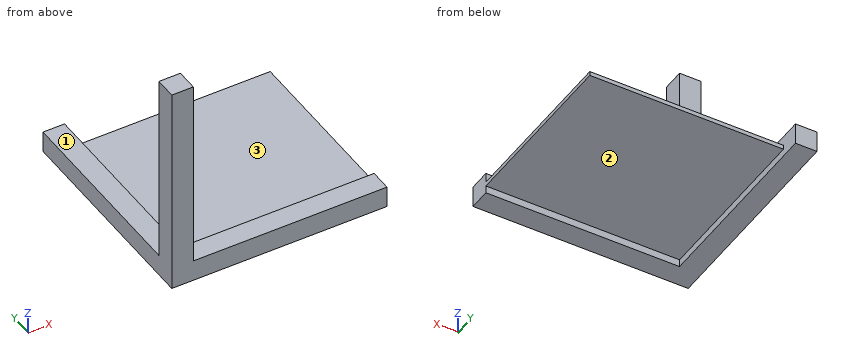
```python
from build123d import *

# Parameters (mm, degrees)
F0_W     = 200
F0_H     = 20
F1_DEPTH = 20
F2_W     = 20
F2_H     = 20
F3_DEPTH = 180
F4_W     = 20
F4_H     = 20
F5_DEPTH = 180
F6_W     = 180
F6_H     = 4
F7_DEPTH = 161.4


with BuildPart() as f1:
    # F0 (on Top) → F1 (new body)
    with BuildSketch(Plane.XY):
        with Locations((100, 10)):
            Rectangle(F0_W, F0_H)
    extrude(amount=F1_DEPTH)

    # F2 (on face) → F3 (join)
    with BuildSketch(Plane.XY.offset(20)):
        with Locations((10, 10)):
            Rectangle(F2_W, F2_H)
    extrude(amount=F3_DEPTH)

    # F4 (on face) → F5 (join)
    with BuildSketch(Plane(origin=(0, 20, 0), x_dir=(-1, 0, 0), z_dir=(0, 1, 0))):
        with Locations((-10, 10)):
            Rectangle(F4_W, F4_H)
    extrude(amount=F5_DEPTH)

    # F6 (on face) → F7 (join)
    with BuildSketch(Plane(origin=(0, 20, 0), x_dir=(-1, 0, 0), z_dir=(0, 1, 0))):
        with Locations((-110, 9)):
            Rectangle(F6_W, F6_H)
    extrude(amount=F7_DEPTH)


solid = f1.part
```
The model under review builds one solid part; all positions refer to its coordinate system, in mm. Face numbers are marked on the shaded views. A direction names the side the tool comes from. Coordinates: 2 decimals unless noted, no trailing zeros. Write each loop counter-clockwise with the first axis right and the second up, starting at its lowest first coordinate (ties: lowest second). Pieces come first, ordered by that corner, then holes. Notation, with made-up numbers: (76.25, 2.5) - (116.25, 2.5) arc R9 cw to (116.25, 12.5) - close; hole circle Ø4 at (80.25, 58). An arc over 180 degrees is marked (long way). Write item = value, one per line.
(1) Consider section D-D, the plane z = 97.5. Give the boundary of the cut face in (x, y).
Result sheet:
outline = (0, 0) - (20, 0) - (20, 20) - (0, 20) - close
(2) Consider section C-C, the plane z = 14.5. Give the boundary of the cut face in (x, y).
Result sheet:
outline = (0, 0) - (200, 0) - (200, 20) - (20, 20) - (20, 200) - (0, 200) - close
(3) Consider section B-B, the plane x = 38. Give the boundary of the cut face in (y, z).
Result sheet:
outline = (0, 0) - (20, 0) - (20, 7) - (181.4, 7) - (181.4, 11) - (20, 11) - (20, 20) - (0, 20) - close
(4) For line 1 (Z direction, x = 188.5, y = 132); line 2 (Z direction, x = 17, y = 137), list the stretches that pass through material, from the lowest coordinate up. Write a range as [from, to].
Result sheet:
line_1 = [7, 11]
line_2 = [0, 20]
(5) Consider section A-A, the plane y = 79. Give the boundary of the cut face in (x, z).
Result sheet:
outline = (0, 0) - (20, 0) - (20, 7) - (200, 7) - (200, 11) - (20, 11) - (20, 20) - (0, 20) - close
(6) Machinability: for the marked faces 1, 2 and 3, which of the approach directions +Z, -Z, +X, -X, +Y, -Y give a long, thin tool a straight path to every point of the face, cutting with its end or side? Answer none if there is none.
Result sheet:
face_1 = +Z, +X, -X, +Y
face_2 = -Z, +X, +Y
face_3 = +Z, +X, +Y
(7) For P1, Ø2, axis at x = 147.5, z = 3.5, coming from the +Y side; P2, Ø3, axis at x = 106.5, z = 8, coming from the +Y side; P3, Ø8, axis at x = 123, y = 20, coming from the -Z side; P4, Ø10, axis at y = 5, z = 134.5, coming from the +X side, all flat-tipped, find the tip position at first contact; note any pin that passes through.
Result sheet:
P1 = 20
P2 = 181.4
P3 = 0
P4 = 20
